```python
from build123d import *

# Parameters (mm, degrees)
F1_DEPTH = 25.4
F2_SIZE  = 5.08
F4_DEPTH = 15.24
F6_DEPTH = 15.24


with BuildPart() as f1:
    # F0 (on Front) → F1 (new body)
    with BuildSketch(Plane.XZ):
        with BuildLine():
            Line((27.518749, 22.430017), (28.481669, 29.77331))
            ThreePointArc((28.481669, 29.77331), (0, 58.254979), (-28.481669, 29.77331))
            Line((-28.481669, 29.77331), (-27.446961, 22.166089))
            ThreePointArc((-27.446961, 22.166089), (0.136758, 1.291969), (27.518749, 22.430017))
        make_face()
        with BuildLine():
            ThreePointArc((27.518749, 22.430017), (28.239913, 26.070231), (28.481669, 29.77331))
            Line((28.481669, 29.77331), (27.518749, 22.430017))
        make_face()
        with BuildLine():
            Line((-27.446961, 22.166089), (-28.481669, 29.77331))
            ThreePointArc((-28.481669, 29.77331), (-28.221807, 25.934676), (-27.446961, 22.166089))
        make_face()
        with BuildLine():
            Line((14.615998, -75.967178), (27.518749, 22.430017))
            ThreePointArc((27.518749, 22.430017), (0.136758, 1.291969), (-27.446961, 22.166089))
            Line((-27.446961, 22.166089), (-14.074668, -76.147616))
            Line((-14.074668, -76.147616), (14.615998, -75.967178))
        make_face()
    extrude(amount=F1_DEPTH)

    # F2
    f2_edges = [f1.edges().sort_by_distance(p)[0] for p in [
        (0.270665, 0, -76.057397),
    ]]
    chamfer(f2_edges, length=F2_SIZE)

    # F3 (on Right) → F4 (join)
    with BuildSketch(Plane.YZ):
        Polygon((54.190729, -75.843684), (0, 0), (0, -75.843684), align=None)
    extrude(amount=F4_DEPTH)

    # F5 (on Right) → F6 (join)
    with BuildSketch(Plane.YZ):
        Polygon((53.829387, -75.629257), (0, 0), (0, -75.629257), align=None)
    extrude(amount=-F6_DEPTH)


solid = f1.part
```
Work out the finished part from the listing and answer in its coordinate system (mm). A direction names the side the tool comes from. Give positions to 0.01 mm unless a question says otherwise; leave off trailing zeros. Loops run counter-clockwise (first coordinate to the right, second up) from the corner with the lowest first, then second, coordinate; pieces in that order, holes last. Notation, with made-up numbers: (-11.5, -3.5) -> (18.5, -3.5) arc R14 cw to (18.5, 2.5) -> close; hole circle Ø1 at (-9, -37). An arc over 180 degrees is marked (long way). Use CSV: the item, a comma, the result in double quotes.
1. The part is cut by section D-D (z = -36). Write down the section's boundary in (x, y).
Found:
outline,"(-19.54, -25.4) -> (19.86, -25.4) -> (19.86, 0) -> (15.24, 0) -> (15.24, 25.72) -> (0, 25.72) -> (0, 25.62) -> (-15.24, 25.62) -> (-15.24, 0) -> (-19.54, 0) -> close"
2. The mould has two halves that part along Y. Classify faces 1 (the flat face through (0, -25.4, -8)), 2 (the flat face through (-7.51, 27.29, -38.34)), 3 (the flat face through (0, 0, -73)): +Y half, -Y half, draft (parallel to the pull), parting line (faces both ways), or undercut.
Found:
face 1,"-Y half"
face 2,"+Y half"
face 3,"undercut"
3. Flat-ended cylindrical pins translate along their axes: pin 1 Ø1 at (x, y) = (-4, 24.5) entering from -Z; pin 2 Ø5 at (x, y) = (17, 38) entering from +Z; pin 3 Ø4 at (x, z) = (-22, -9) entering from +Y. Find the tip coordinate at first contact, or state that the pin passes through.
Found:
pin 1,"z = -75.63"
pin 2,"z = -50.7"
pin 3,"y = 0"
4. A tool of negligible diameter and unlimited length cuts with its end or side. For faces 4 (the flat face through (-8, 27, -75.629)), 5 (the flat face through (15.24, 15, -54)), 6 (the flat face through (-15.24, 15, -54)), from which of +Z, -Z, +X, -X, +Y, -Y can it reach the whole face along a straight path? Write none if from no direction.
Found:
face 4,"-Z, -X, +Y"
face 5,"+Z, -Z, +X, +Y"
face 6,"+Z, -Z, -X, +Y"
5. Straight lines are drawn through the part: line 1 (Y direction, x = 17, z = 23.5); line 2 (Y direction, x = -10, z = -31.5); line 3 (X direction, y = 9.5, z = -50.5). For each, find the intervals that lie inside material, in ascending order.
Found:
line 1,"-25.4 to 0"
line 2,"-25.4 to 22.42"
line 3,"-15.24 to 15.24"
6. The part is cut by section C-C (x = 6). Write down the section's boundary in (y, z).
Found:
outline,"(-25.4, -76.02) -> (-5.08, -76.02) -> (0, -70.94) -> (0, -75.84) -> (54.19, -75.84) -> (0, 0) -> (0, 57.62) -> (-25.4, 57.62) -> close"
7. The part is cut by section A-A (y = 27). Write down the section's boundary in (x, z).
Found:
outline,"(-15.24, -75.63) -> (0, -75.63) -> (0, -75.84) -> (15.24, -75.84) -> (15.24, -37.79) -> (0, -37.79) -> (0, -37.93) -> (-15.24, -37.93) -> close"
8. The part is cut by section B-B (z = -59.5). Write down the section's boundary in (x, y), then the cut area to 3 significant figures.
Found:
outline,"(-16.34, -25.4) -> (16.78, -25.4) -> (16.78, 0) -> (15.24, 0) -> (15.24, 42.51) -> (0, 42.51) -> (0, 42.35) -> (-15.24, 42.35) -> (-15.24, 0) -> (-16.34, 0) -> close"
area,"2,130 mm^2"
